Can you work these out from the model? Positions are in its coordinate system, mm. A direction names the side the tool comes from. Coordinates: 2 decimals unless noted, no trailing zeros. Order: outer loops, then holes, each group sorted by start corner. A loop starts at its lowest first (then second) coordinate and runs counter-clockwise, first axis right, second up. Notation, with made-up numbers: (39.25, 8.5) -> (61.25, 8.5) arc R29 cw to (61.25, 40.5) -> close; hole circle Ø7 at (-12, 32.25). An arc over 180 degrees is marked (long way). Use a Markdown table: item, result. Add a question column.
1. If I drill on line 1 along X through (y, z) = (4.75, 0); line 2 along Z through (x, y) = (-6.35, 3.5); line 3 along X through (y, z) = (1.25, -0.5), over which ranges is the centre line in solid material (lowest first)? Write a range as from..to.
2. Suppose I cut it at B-B, the plane z = 0. List the corners of the cut face in (x, y) for me, then the cut area to 3 significant figures.
3. For faces 4 (the flat face through (-6, 3, 3.556)), 5 (the flat face through (-50.71, 3.13, 14.42)), 6 (the flat face through (-25.31, 3.13, 14.58)), which set-ups out of +Z, -Z, +X, -X, +Y, -Y let a thin tool reach every point of the face, with its end or its side?
4. Suppose I cut it at A-A, the plane x = -6.35. List the corners of the cut face in (y, z) for me.
5. Suppose I cut it at D-D, the plane x = -30.5. List the corners of the cut face in (y, z) for me.
6. For pin 1 Ø1.8 at (x, z) = (-2.54, 0) entering from +Y; pin 2 Ø3 at (x, y) = (-11.5, 2.5) entering from +Z, each with a flat end and sliding along its axis, tell me the tip position at first contact or that it passes through.
7. We'd pull the mould along Z, two halves only. Please class faces 1 (the flat face through (-27, 6.35, 8)), 2 (the flat face through (-28.8, 3.13, 4.17)), 3 (the cylindrical face through (-1.484, 3.131, 0.438)): pulls with the +Z half, pulls with the -Z half, needs draft (parallel to the pull), parting line crosses it, or undercut.
8. Suppose I cut it at C-C, the plane y = 2.5. List the corners of the cut face in (x, z) for me.
```python
from build123d import *

# Parameters (mm, degrees)
SKETCH2_W           = 12.7
SKETCH2_H           = 7.112
SKETCH2_R           = 1.143
BOSS_EXTRUDE1_DEPTH = 6.35
BOSS_EXTRUDE2_DEPTH = 6.35


with BuildPart() as part:
    # Sketch2 → Boss-Extrude1 (new body)
    with BuildSketch(Plane(origin=(0, 0, 0), x_dir=(1, 0, 0), z_dir=(0, 1, 0))):
        Polygon((-12.7, -3.556), (-31.75, -11.684), (-44.45, -11.684), (-12.7, 3.556), align=None)
        with Locations((-6.35, 0)):
            Rectangle(SKETCH2_W, SKETCH2_H)
        with Locations((-6.35, 0)):
            Circle(SKETCH2_R, mode=Mode.SUBTRACT)
        with Locations((-2.54, 0)):
            Circle(SKETCH2_R, mode=Mode.SUBTRACT)
    extrude(amount=BOSS_EXTRUDE1_DEPTH)

    # Sketch3 → Boss-Extrude2 (add)
    with BuildSketch(Plane(origin=(0, 0, 0), x_dir=(1, 0, 0), z_dir=(0, 1, 0))):
        Polygon((-44.45, -11.684), (-57.15, -17.231593434), (-19.05, -17.3978371), (-31.75, -11.684), align=None)
    extrude(amount=BOSS_EXTRUDE2_DEPTH)


solid = part.part
```
Worked out:
| question | item | result |
|---|---|---|
| 1 | line 1 | x = -20.11..-7.49, -5.21..-3.68, -1.4..0 |
| 1 | line 2 | z = -3.56..-1.14, 1.14..3.56 |
| 1 | line 3 | x = -19.07..-7.38, -5.32..-3.57, -1.51..0 |
| 2 | outline | (-20.11, 0) -> (-7.49, 0) -> (-7.49, 6.35) -> (-20.11, 6.35) -> close; (-5.21, 0) -> (-3.68, 0) -> (-3.68, 6.35) -> (-5.21, 6.35) -> close; (-1.4, 0) -> (0, 0) -> (0, 6.35) -> (-1.4, 6.35) -> close |
| 2 | area | 98.7 mm² |
| 3 | face 4 | +Z, +X, +Y, -Y |
| 3 | face 5 | -Z, -X, +Y, -Y |
| 3 | face 6 | +X, +Y, -Y |
| 4 | outline | (0, -3.56) -> (6.35, -3.56) -> (6.35, -1.14) -> (0, -1.14) -> close; (0, 1.14) -> (6.35, 1.14) -> (6.35, 3.56) -> (0, 3.56) -> close |
| 5 | outline | (0, 4.99) -> (6.35, 4.99) -> (6.35, 11.15) -> (0, 11.15) -> close; (0, 12.25) -> (6.35, 12.25) -> (6.35, 17.35) -> (0, 17.35) -> close |
| 6 | pin 1 | passes through |
| 6 | pin 2 | stops at z = 3.68 |
| 7 | face 1 | needs draft |
| 7 | face 2 | pulls with the -Z half |
| 7 | face 3 | undercut |
| 8 | outline | (-57.15, 17.23) -> (-44.45, 11.68) -> (-12.7, -3.56) -> (0, -3.56) -> (0, 3.56) -> (-12.7, 3.56) -> (-31.75, 11.68) -> (-19.05, 17.4) -> close; hole circle Ø2.29 at (-6.35, 0); hole circle Ø2.29 at (-2.54, 0) |
